Here's how the part is built. I have some questions about the finished solid (model axes, mm). Round coordinates to 2 decimals unless told otherwise and drop trailing zeros. Loops run counter-clockwise (first coordinate to the right, second up) from the corner with the lowest first, then second, coordinate; pieces in that order, holes last. Notation, with made-up numbers: M 20,70 L 33,70 A22 cw 33,86 Z; hole C 64,72 d1. An arc over 180 degrees is marked long. Answer as CSV lines item,"result".
```python
from build123d import *

# Parameters (mm, degrees)
F0_W     = 396
F0_H     = 100
F0_R     = 1.13
F1_DEPTH = 5


with BuildPart() as f1:
    # F0 (on Top) → F1 (new body)
    with BuildSketch(Plane.XY):
        Rectangle(F0_W, F0_H)
        with Locations((-99, -47.25)):
            Circle(F0_R, mode=Mode.SUBTRACT)
        with Locations((0, -47.25)):
            Circle(F0_R, mode=Mode.SUBTRACT)
        with Locations((99, -47.25)):
            Circle(F0_R, mode=Mode.SUBTRACT)
        with BuildLine():
            ThreePointArc((-182, 29), (-180.535534, 32.535534), (-177, 34))
            Line((-177, 34), (-72, 34))
            ThreePointArc((-72, 34), (-68.464466, 32.535534), (-67, 29))
            Line((-67, 29), (-67, -29))
            ThreePointArc((-67, -29), (-68.464466, -32.535534), (-72, -34))
            Line((-72, -34), (-177, -34))
            ThreePointArc((-177, -34), (-180.535534, -32.535534), (-182, -29))
            Line((-182, -29), (-182, 29))
        make_face(mode=Mode.SUBTRACT)
        with Locations((-99, 47.25)):
            Circle(F0_R, mode=Mode.SUBTRACT)
        with BuildLine():
            ThreePointArc((67, 29), (68.464466, 32.535534), (72, 34))
            Line((72, 34), (177, 34))
            ThreePointArc((177, 34), (180.535534, 32.535534), (182, 29))
            Line((182, 29), (182, -29))
            ThreePointArc((182, -29), (180.535534, -32.535534), (177, -34))
            Line((177, -34), (72, -34))
            ThreePointArc((72, -34), (68.464466, -32.535534), (67, -29))
            Line((67, -29), (67, 29))
        make_face(mode=Mode.SUBTRACT)
        with Locations((0, 47.25)):
            Circle(F0_R, mode=Mode.SUBTRACT)
        with Locations((99, 47.25)):
            Circle(F0_R, mode=Mode.SUBTRACT)
    extrude(amount=F1_DEPTH)


solid = f1.part
```
1. I want a section at C-C, the plane z = 3. Count the separate pieces of the cut face and the enclosed holes in it, and give its area (3 significant figures).
Evaluation:
separate pieces,"1"
enclosed holes,"8"
area,"24,000 mm²"
2. If I drill on line 1 (X direction, y = 18, z = 3.2); line 2 (Y direction, x = 99, z = 2.4); line 3 (Y direction, x = -82, z = 1.75), over which ranges is the centre line in solid material (lowest first)? Write a range as [from, to].
Evaluation:
line 1,"x = [-198, -182], [-67, 67], [182, 198]"
line 2,"y = [-50, -48.38], [-46.12, -34], [34, 46.12], [48.38, 50]"
line 3,"y = [-50, -34], [34, 50]"
3. I want a section at B-B, the plane y = -8. Please give me the cut outline in (x, z), and give its area (3 significant figures).
Evaluation:
outline,"M -198,0 L -182,0 L -182,5 L -198,5 Z; M -67,0 L 67,0 L 67,5 L -67,5 Z; M 182,0 L 198,0 L 198,5 L 182,5 Z"
area,"830 mm²"
4. I want a section at A-A, the plane x = 165. Please give me the cut outline in (y, z).
Evaluation:
outline,"M -50,0 L -34,0 L -34,5 L -50,5 Z; M 34,0 L 50,0 L 50,5 L 34,5 Z"
